from build123d import *

# Parameters (mm, degrees)
SKETCH1_W           = 1524
SKETCH1_H           = 1524
BOSS_EXTRUDE1_DEPTH = 127
SKETCH2_R           = 254
BOSS_EXTRUDE2_DEPTH = 1092.2
SKETCH3_R           = 317.5
BOSS_EXTRUDE3_DEPTH = 177.8
FILLET1_R           = 254


with BuildPart() as part:
    # Sketch1 → Boss-Extrude1 (new body)
    with BuildSketch(Plane.XY):
        Rectangle(SKETCH1_W, SKETCH1_H)
    extrude(amount=BOSS_EXTRUDE1_DEPTH)

    # Sketch2 → Boss-Extrude2 (add)
    with BuildSketch(Plane.XY.offset(127)):
        Circle(SKETCH2_R)
    extrude(amount=BOSS_EXTRUDE2_DEPTH)

    # Sketch3 → Boss-Extrude3 (add)
    with BuildSketch(Plane.XY.offset(127)):
        with Locations(Location((0, 0, 0), (0, 0, 180))):
            Circle(SKETCH3_R)
    extrude(amount=BOSS_EXTRUDE3_DEPTH)

    # Fillet1
    fillet1_edges = [part.edges().sort_by_distance(p)[0] for p in [
        (-762, 762, 63.5),
        (762, 762, 63.5),
    ]]
    fillet(fillet1_edges, radius=FILLET1_R)


solid = part.part
Can you work these out from the model? Positions are in its coordinate system, mm. A direction names the side the tool comes from. Round coordinates to 2 decimals unless told otherwise and drop trailing zeros. Loops run counter-clockwise (first coordinate to the right, second up) from the corner with the lowest first, then second, coordinate; pieces in that order, holes last. Notation, with made-up numbers: (64, 64) - (74, 64) arc R25 ccw to (74, 81) - close; hole circle Ø10 at (2, 78). An arc over 180 degrees is marked (long way). Write item = value, one per line. Start each with the question number.
(1) If we section it at D-D (y = -529): Please give me the cut outline in (x, z), and give its area (3 significant figures).
(2) If we section it at C-C (z = 530): Please give me the cut outline in (x, y).
(3) If I drill on probe 1 along Z at (x, y) = (290, -249.5); probe 2 along Y at (x, z) = (520, 119); probe 3 along X at (y, z) = (196, 133), over which ranges is the centre line in solid material (lowest first)? Write a range as [from, to].
(4) For P1, Ø2, axis at x = 201, y = 312, coming from the +Z side; P2, Ø8, axis at y = 122.5, z = 1055.5, coming from the -X side, each with a flat end and sliding along its axis, tell me the tip position at first contact or that it passes through.
(5) If we section it at A-A (x = 0): Please give me the cut outline in (y, z), and give its area (3 significant figures).
(6) For faces 1 (the face through (762, -136, 63)), 2 (the face through (328, 11, 127)), which set-ups out of +Z, -Z, +X, -X, +Y, -Y let a thin tool reach every point of the face, with its end or its side?
Ans:
q1.outline = (-762, 0) - (762, 0) - (762, 127) - (-762, 127) - close
q1.area = 194,000 mm²
q2.outline = circle Ø508 at (0, 0)
q3.probe_1 = [0, 127]
q3.probe_2 = [-762, 761.72]
q3.probe_3 = [-249.78, 249.78]
q4.P1 = 127
q4.P2 = -224.66
q5.outline = (-762, 0) - (762, 0) - (762, 127) - (317.5, 127) - (317.5, 304.8) - (254, 304.8) - (254, 1219.2) - (-254, 1219.2) - (-254, 304.8) - (-317.5, 304.8) - (-317.5, 127) - (-762, 127) - close
q5.area = 771,000 mm²
q6.face_1 = +Z, -Z, +X, +Y, -Y
q6.face_2 = +Z
